Input: part model. Units: mm. Frame: model coordinates. Round coordinates to 2 decimals unless told otherwise and drop trailing zeros. Order: outer loops, then holes, each group sorted by start corner. A loop starts at its lowest first (then second) coordinate and runs counter-clockwise, first axis right, second up. Notation, with made-up numbers: (-19, -32) -> (-9, -32) arc R19 cw to (-9, -10) -> close; hole circle Ø8 at (42.5, 6). An arc over 180 degrees is marked (long way). Use a Markdown table: item, result.
from build123d import *

# Parameters (mm, degrees)
F1_START = 69
F0_R     = 2.5
F1_DEPTH = 10
F2_R     = 5


with BuildPart() as f1:
    # F0 (on Top) → F1 (new body)
    with BuildSketch(Plane.XY.offset(F1_START)):
        with BuildLine():
            Line((28.115, 28.115), (-28.115, 28.115))
            Line((-28.115, 28.115), (-28.115, 7.6560907126))
            ThreePointArc((-28.115, 7.6560907126), (-22.7514332101, 7.7037324483), (-18.5240804258, 4.4022771811))
            ThreePointArc((-18.5240804258, 4.4022771811), (0, 19.04), (18.5240804258, 4.4022771811))
            ThreePointArc((18.5240804258, 4.4022771811), (22.7514332101, 7.7037324483), (28.115, 7.6560907126))
            Line((28.115, 7.6560907126), (28.115, 28.115))
        make_face()
        with Locations((-23.62, 23.62)):
            Circle(F0_R, mode=Mode.SUBTRACT)
        with Locations((23.62, 23.62)):
            Circle(F0_R, mode=Mode.SUBTRACT)
        with BuildLine():
            ThreePointArc((-18.5240804258, 4.4022771811), (-22.7514332101, 7.7037324483), (-28.115, 7.6560907126))
            Line((-28.115, 7.6560907126), (-28.115, 2.0247777656))
            ThreePointArc((-28.115, 2.0247777656), (-24.2994074418, 3.2444934119), (-21.95, 0))
            ThreePointArc((-21.95, 0), (-24.2994074418, -3.2444934119), (-28.115, -2.0247777656))
            Line((-28.115, -2.0247777656), (-28.115, -7.6560907126))
            ThreePointArc((-28.115, -7.6560907126), (-22.7514332101, -7.7037324483), (-18.5240804258, -4.4022771811))
            ThreePointArc((-18.5240804258, -4.4022771811), (-19.04, 0), (-18.5240804258, 4.4022771811))
        make_face()
        with BuildLine():
            ThreePointArc((-21.95, 0), (-24.2994074418, 3.2444934119), (-28.115, 2.0247777656))
            Line((-28.115, 2.0247777656), (-28.115, -2.0247777656))
            ThreePointArc((-28.115, -2.0247777656), (-24.2994074418, -3.2444934119), (-21.95, 0))
        make_face()
        with BuildLine():
            ThreePointArc((-18.5240804258, -4.4022771811), (-22.7514332101, -7.7037324483), (-28.115, -7.6560907126))
            Line((-28.115, -7.6560907126), (-28.115, -28.115))
            Line((-28.115, -28.115), (-7.6560907126, -28.115))
            ThreePointArc((-7.6560907126, -28.115), (-7.7037324483, -22.7514332101), (-4.4022771811, -18.5240804258))
            ThreePointArc((-4.4022771811, -18.5240804258), (-13.4633131138, -13.4633131138), (-18.5240804258, -4.4022771811))
        make_face()
        with Locations((-23.62, -23.62)):
            Circle(F0_R, mode=Mode.SUBTRACT)
        with BuildLine():
            ThreePointArc((4.4022771811, -18.5240804258), (0, -19.04), (-4.4022771811, -18.5240804258))
            ThreePointArc((-4.4022771811, -18.5240804258), (-7.7037324483, -22.7514332101), (-7.6560907126, -28.115))
            Line((-7.6560907126, -28.115), (-2.0247777656, -28.115))
            ThreePointArc((-2.0247777656, -28.115), (-1.5407155692, -22.3173089831), (3.415, -25.365))
            ThreePointArc((3.415, -25.365), (3.0476910169, -26.9057155692), (2.0247777656, -28.115))
            Line((2.0247777656, -28.115), (7.6560907126, -28.115))
            ThreePointArc((7.6560907126, -28.115), (8.0143784209, -26.7606946394), (8.135, -25.365))
            ThreePointArc((8.135, -25.365), (7.1411046018, -21.4684823155), (4.4022771811, -18.5240804258))
        make_face()
        with BuildLine():
            ThreePointArc((3.415, -25.365), (-1.5407155692, -22.3173089831), (-2.0247777656, -28.115))
            Line((-2.0247777656, -28.115), (2.0247777656, -28.115))
            ThreePointArc((2.0247777656, -28.115), (3.0476910169, -26.9057155692), (3.415, -25.365))
        make_face()
        with BuildLine():
            Line((28.115, -28.115), (28.115, -7.6560907126))
            ThreePointArc((28.115, -7.6560907126), (22.7514332101, -7.7037324483), (18.5240804258, -4.4022771811))
            ThreePointArc((18.5240804258, -4.4022771811), (13.4633131138, -13.4633131138), (4.4022771811, -18.5240804258))
            ThreePointArc((4.4022771811, -18.5240804258), (7.1411046018, -21.4684823155), (8.135, -25.365))
            ThreePointArc((8.135, -25.365), (8.0143784209, -26.7606946394), (7.6560907126, -28.115))
            Line((7.6560907126, -28.115), (28.115, -28.115))
        make_face()
        with Locations((23.62, -23.62)):
            Circle(F0_R, mode=Mode.SUBTRACT)
        with BuildLine():
            Line((28.115, 2.0247777656), (28.115, 7.6560907126))
            ThreePointArc((28.115, 7.6560907126), (22.7514332101, 7.7037324483), (18.5240804258, 4.4022771811))
            ThreePointArc((18.5240804258, 4.4022771811), (18.9105802569, 2.2162026862), (19.04, 0))
            ThreePointArc((19.04, 0), (18.9105802569, -2.2162026862), (18.5240804258, -4.4022771811))
            ThreePointArc((18.5240804258, -4.4022771811), (22.7514332101, -7.7037324483), (28.115, -7.6560907126))
            Line((28.115, -7.6560907126), (28.115, -2.0247777656))
            ThreePointArc((28.115, -2.0247777656), (21.95, 0), (28.115, 2.0247777656))
        make_face()
        with BuildLine():
            Line((28.115, -2.0247777656), (28.115, 2.0247777656))
            ThreePointArc((28.115, 2.0247777656), (21.95, 0), (28.115, -2.0247777656))
        make_face()
    extrude(amount=F1_DEPTH)

    # F2
    f2_edges = [f1.edges().sort_by_distance(p)[0] for p in [
        (-28.115, -28.115, 74),
        (-28.115, 28.115, 74),
        (28.115, 28.115, 74),
        (28.115, -28.115, 74),
    ]]
    fillet(f2_edges, radius=F2_R)


solid = f1.part
1) Cut plane B-B on y = -15. Return loops of the section in (x, z) (3 decimals).
Results found:
| item | result |
|---|---|
| outline | (-28.115, 69) -> (-11.727, 69) -> (-11.727, 79) -> (-28.115, 79) -> close; (11.727, 69) -> (28.115, 69) -> (28.115, 79) -> (11.727, 79) -> close |
2) Cut plane D-D on y = 22. Return loops of the section in (x, z) (3 decimals), and give its area (3 significant figures).
Results found:
| item | result |
|---|---|
| outline | (-28.115, 69) -> (-25.524, 69) -> (-25.524, 79) -> (-28.115, 79) -> close; (-21.716, 69) -> (21.716, 69) -> (21.716, 79) -> (-21.716, 79) -> close; (25.524, 69) -> (28.115, 69) -> (28.115, 79) -> (25.524, 79) -> close |
| area | 486 mm² |
3) Pin query (flat end, axial travel): pin 1 Ø6 at (x, y) = (-23.62, 23.62) entering from +Z. Return the tip coordinate at first contact, or that it passes through.
Results found:
| item | result |
|---|---|
| pin 1 | stops at z = 79 |
4) Line query: L1, parallel to X at y = 23.5, z = 70.25; L2, parallel to Y at x = -23.62, z = 76.5; L3, parallel to X at y = 0, z = 70.75 (3 decimals). Output: solid intervals per line, ascending. Write a range as [from, to].
Results found:
| item | result |
|---|---|
| L1 | x = [-28.1, -26.12], [-21.12, 21.12], [26.12, 28.1] |
| L2 | y = [-28.09, -26.12], [-21.12, 21.12], [26.12, 28.09] |
| L3 | x = [-28.115, -19.04], [19.04, 28.115] |
5) Cut plane C-C on z = 70. Return loops of the section in (x, y) (3 decimals).
Results found:
| item | result |
|---|---|
| outline | (-28.115, -23.115) arc R5 ccw to (-23.115, -28.115) -> (23.115, -28.115) arc R5 ccw to (28.115, -23.115) -> (28.115, 23.115) arc R5 ccw to (23.115, 28.115) -> (-23.115, 28.115) arc R5 ccw to (-28.115, 23.115) -> close; hole circle Ø5 at (-23.62, -23.62); hole circle Ø5 at (-23.62, 23.62); hole circle Ø38.08 at (0, 0); hole circle Ø5 at (23.62, -23.62); hole circle Ø5 at (23.62, 23.62) |
6) Cut plane A-A on x = -9. Return loops of the section in (y, z) (3 decimals).
Results found:
| item | result |
|---|---|
| outline | (-28.115, 69) -> (-16.779, 69) -> (-16.779, 79) -> (-28.115, 79) -> close; (16.779, 69) -> (28.115, 69) -> (28.115, 79) -> (16.779, 79) -> close |
7) Pull-direction query (Y, two-part tool) for faces 1 (the cylindrical face through (-22.28, -21.51, 73.93)), 2 (the cylindrical face through (24.96, -21.51, 73.93)), 3 (the flat face through (-28.115, 0, 74)), 4 (the cylindrical face through (-26.7, -26.6, 74.1)); classes: +Y half, -Y half, draft (parallel to the pull), parting line (faces both ways), or undercut.
Results found:
| item | result |
|---|---|
| face 1 | undercut |
| face 2 | undercut |
| face 3 | draft |
| face 4 | -Y half |
